from build123d import *

# Parameters (mm, degrees)
F1_DEPTH = 40
F2_DEPTH = 24
F4_DEPTH = 10
F5_DEPTH = 30.001


with BuildPart() as f1:
    # F0 (on Right) → F1 (new body, symmetric)
    with BuildSketch(Plane.YZ):
        Polygon((-100, 0), (0, 0), (0, 30), (-44, 30), (-100, 30), align=None)
        with BuildLine():
            Line((-44, 30), (0, 30))
            Line((0, 30), (0, 68))
            ThreePointArc((0, 68), (-22, 46), (-44, 68))
            Line((-44, 68), (-44, 30))
        make_face()
        with BuildLine():
            ThreePointArc((-44, 68), (-22, 46), (0, 68))
            Line((0, 68), (-12, 68))
            ThreePointArc((-12, 68), (-22, 58), (-32, 68))
            Line((-32, 68), (-44, 68))
        make_face()
        with BuildLine():
            Line((-12, 68), (0, 68))
            ThreePointArc((0, 68), (-22, 90), (-44, 68))
            Line((-44, 68), (-32, 68))
            ThreePointArc((-32, 68), (-22, 78), (-12, 68))
        make_face()
    extrude(amount=F1_DEPTH, both=True)

    # F0 (on Right) → F2 (cut, symmetric)
    with BuildSketch(Plane.YZ):
        with BuildLine():
            Line((-44, 30), (0, 30))
            Line((0, 30), (0, 68))
            ThreePointArc((0, 68), (-22, 46), (-44, 68))
            Line((-44, 68), (-44, 30))
        make_face()
        with BuildLine():
            ThreePointArc((-44, 68), (-22, 46), (0, 68))
            Line((0, 68), (-12, 68))
            ThreePointArc((-12, 68), (-22, 58), (-32, 68))
            Line((-32, 68), (-44, 68))
        make_face()
        with BuildLine():
            Line((-12, 68), (0, 68))
            ThreePointArc((0, 68), (-22, 90), (-44, 68))
            Line((-44, 68), (-32, 68))
            ThreePointArc((-32, 68), (-22, 78), (-12, 68))
        make_face()
        with BuildLine():
            Line((-32, 68), (-12, 68))
            ThreePointArc((-12, 68), (-22, 78), (-32, 68))
        make_face()
    extrude(amount=F2_DEPTH, both=True, mode=Mode.SUBTRACT)

    # F3 (on face) → F4 (cut)
    with BuildSketch(Plane.XY.offset(30)):
        with BuildLine():
            Line((16, -100), (16, -83.1376686692))
            ThreePointArc((16, -83.1376686692), (0, -67.1376686692), (-16, -83.1376686692))
            Line((-16, -83.1376686692), (-16, -100))
            Line((-16, -100), (-8, -100))
            Line((-8, -100), (-8, -83.1376686692))
            ThreePointArc((-8, -83.1376686692), (0, -75.1376686692), (8, -83.1376686692))
            Line((8, -83.1376686692), (8, -100))
            Line((8, -100), (16, -100))
        make_face()
    extrude(amount=-F4_DEPTH, mode=Mode.SUBTRACT)

    # F5 (cut, through all): a face of the model
    f5_faces = [f1.faces().sort_by_distance(p)[0] for p in [
        (0, -88.3583676716, 30),
    ]]
    extrude(f5_faces, amount=-F5_DEPTH, mode=Mode.SUBTRACT)


solid = f1.part
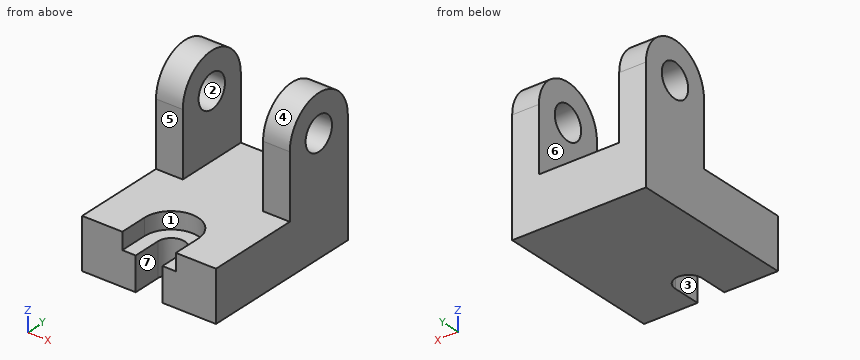
Can you work these out from the model? Positions are in its coordinate system, mm. Face numbers are marked on the shaded views. A direction names the side the tool comes from. Round coordinates to 2 decimals unless told otherwise and drop trailing zeros. Loops run counter-clockwise (first coordinate to the right, second up) from the corner with the lowest first, then second, coordinate; pieces in that order, holes last. Notation, with made-up numbers: (85.5, -13) - (110.5, -13) arc R27 ccw to (110.5, 9) - close; hole circle Ø6 at (78, 61.5). An arc over 180 degrees is marked (long way). Answer in a Markdown table with one row per item. Add a question column.
Q1. For pin 1 Ø5 at (x, y) = (-10.5, -72.5) entering from +Z; pin 2 Ø22 at (y, z) = (-22, 71) entering from -X; pin 3 Ø13 at (x, z) = (32, 47) entering from -Y; pin 4 Ø12 at (y, z) = (-22, 68) entering from -X, each with a flat end and sliding along its axis, tell me the tip position at first contact or that it passes through.
Q2. I want a section at A-A on y = -22. List the corners of the cut face in (x, z) for me.
Q3. I want a section at B-B on z = 36.5. List the corners of the cut face in (x, y) for me.
Q4. I need wall thicknesses on L1, parallel to Z at x = 32, y = -22; L2, parallel to Y at x = 29.25, z = 68; L3, parallel to X at y = -41.5, z = 36. Which ranges of each line are inside material? Lowest first, please.
Q5. I want a section at C-C on x = -34. List the corners of the cut face in (y, z) for me, and give its area (3 significant figures).
Q6. We'd pull the mould along Y, two halves only. Please class the marked faces 1, 2, 3 and 4: pulls with the +Y half, pulls with the -Y half, needs draft (parallel to the pull), parting line crosses it, or undercut.
Q7. I want a section at D-D on z = 65. List the corners of the cut face in (x, y) for me, and give its area (3 significant figures).
Q8. Which directions (+Z, -Z, +X, -X, +Y, -Y) give clear straight access to the entire face, cutting with the end or side of a thin tool? Please do the marked faces 5, 6 and 7.
A:
| question | item | result |
|---|---|---|
| 1 | pin 1 | z = 30 |
| 1 | pin 2 | x = -40 |
| 1 | pin 3 | y = -44 |
| 1 | pin 4 | through |
| 2 | outline | (-40, 0) - (40, 0) - (40, 58) - (24, 58) - (24, 30) - (-24, 30) - (-24, 58) - (-40, 58) - close; (-40, 78) - (-24, 78) - (-24, 90) - (-40, 90) - close; (24, 78) - (40, 78) - (40, 90) - (24, 90) - close |
| 3 | outline | (-40, -44) - (-24, -44) - (-24, 0) - (-40, 0) - close; (24, -44) - (40, -44) - (40, 0) - (24, 0) - close |
| 4 | L1 | 0 to 58, 78 to 90 |
| 4 | L2 | -44 to -32, -12 to 0 |
| 4 | L3 | -40 to -24, 24 to 40 |
| 5 | outline | (-100, 0) - (0, 0) - (0, 68) arc R22 ccw to (-44, 68) - (-44, 30) - (-100, 30) - close; hole circle Ø20 at (-22, 68) |
| 5 | area | 5,120 mm^2 |
| 6 | face 1 | pulls with the -Y half |
| 6 | face 2 | undercut |
| 6 | face 3 | needs draft |
| 6 | face 4 | parting line crosses it |
| 7 | outline | (-40, -44) - (-24, -44) - (-24, -31.54) - (-40, -31.54) - close; (-40, -12.46) - (-24, -12.46) - (-24, 0) - (-40, 0) - close; (24, -44) - (40, -44) - (40, -31.54) - (24, -31.54) - close; (24, -12.46) - (40, -12.46) - (40, 0) - (24, 0) - close |
| 7 | area | 797 mm^2 |
| 8 | face 5 | +Z, +X, -X, -Y |
| 8 | face 6 | +Z, +Y, -Y |
| 8 | face 7 | +Z, -Z, -Y |
